Build history of the part. All positions in model axes, mm. A direction names the side the tool comes from. Give positions to 0.01 mm unless a question says otherwise; leave off trailing zeros. Loops run counter-clockwise (first coordinate to the right, second up) from the corner with the lowest first, then second, coordinate; pieces in that order, holes last.
1) Two-plate mould, pull along X, no slides. Class faces 1 (the cylindrical face through (23.09, -9.58, -15.04)), 2 (the flat face through (39, 0, -16)), 3 (the cylindrical face through (20.159, 25.743, -9.706)): +X half, -X half, draft (parallel to the pull), parting line (faces both ways), or undercut.
2) Band-saw the part on C-C on x = 46. List the corners of the cut face in (y, z).
3) Wall check: line 1 (Y direction, x = 0, z = -15.1); line 2 (Y direction, x = 0, z = -13.85); line 3 (X direction, y = -50, z = -14.75). Give the ranges that are in metal, low to high.
4) Band-saw the part on A-A on y = 0. List the corners of the cut face in (x, z).
5) Flat gauge pins, fed straight in: P1, Ø2, axis at x = 21, y = 33, coming from the -Z side; P2, Ø1.2, axis at y = -39.5, z = -15, coming from the +X side; P3, Ø8, axis at y = 41, z = -2, coming from the +X side; P4, Ø7, axis at x = 22.5, y = 22.5, coming from the +Z side. Where does each tip first touch, or does it go through?
6) 3-axis set-ups, long thin cutter, end or side, ignore diameter. For faces 4 (the flat face through (-21, 33, 0)), 5 (the conical face through (24.74, 7.79, -11.75)), 6 (the cylindrical face through (-8.67, -39.05, -4.06)): which of +Z, -Z, +X, -X, +Y, -Y reach the whole face in a straight line?
```python
from build123d import *

# Parameters (mm, degrees)
CYLINDER004_R     = 23.5
CYLINDER004_DEPTH = 6
CYLINDER003_R     = 25
CYLINDER003_DEPTH = 6
CYLINDER_R        = 4
CYLINDER_DEPTH    = 10
CYLINDER005_R     = 25
CYLINDER005_DEPTH = 6
BOX_W             = 110
BOX_H             = 18
BOX_DEPTH         = 1.5
BOX001_W          = 18
BOX001_H          = 110
BOX001_DEPTH      = 1.5
CYLINDER002_R     = 38.5
CYLINDER002_DEPTH = 8
CYLINDER001_R     = 40
CYLINDER001_DEPTH = 8


with BuildPart() as cilindro004:
    # Cylinder004 → Cylinder004 (new body)
    with BuildSketch(Plane.XY.offset(-18)):
        Circle(CYLINDER004_R)
    extrude(amount=CYLINDER004_DEPTH)


with BuildPart() as cut002:
    # Cylinder003 → Cylinder003 (new body)
    with BuildSketch(Plane.XY.offset(-18)):
        Circle(CYLINDER003_R)
    extrude(amount=CYLINDER003_DEPTH)

    # Cut002: cut Cilindro004
    add(cilindro004.part, mode=Mode.SUBTRACT)


with BuildPart() as cilindro:
    # Cylinder → Cylinder (new body)
    with BuildSketch(Plane(origin=(22.5, 22.5, -14), x_dir=(1, 0, 0), z_dir=(0, 0, 1))):
        Circle(CYLINDER_R)
    extrude(amount=CYLINDER_DEPTH)


with BuildPart() as cono001:
    # Cone001 → Cone001 (revolve)
    with BuildSketch(Plane(origin=(0, 0, -12), x_dir=(1, 0, 0), z_dir=(0, -1, 0))):
        Polygon((0, 0), (23.5, 0), (38.5, 4), (0, 4), align=None)
    revolve(axis=Axis((0, 0, -12), (0, 0, 1)))


with BuildPart() as cut004:
    # Cone → Cone (revolve)
    with BuildSketch(Plane(origin=(0, 0, -12), x_dir=(1, 0, 0), z_dir=(0, -1, 0))):
        Polygon((0, 0), (25, 0), (40, 4), (0, 4), align=None)
    revolve(axis=Axis((0, 0, -12), (0, 0, 1)))

    # Cut001: cut Cono001
    add(cono001.part, mode=Mode.SUBTRACT)

    # Cut004: cut Cilindro
    add(cilindro.part, mode=Mode.SUBTRACT)


with BuildPart() as cilindro005:
    # Cylinder005 → Cylinder005 (new body)
    with BuildSketch(Plane.XY.offset(-18)):
        Circle(CYLINDER005_R)
    extrude(amount=CYLINDER005_DEPTH)


with BuildPart() as cubo:
    # Box → Box (new body)
    with BuildSketch(Plane(origin=(-55, -9, 0), x_dir=(1, 0, 0), z_dir=(0, 0, 1))):
        with Locations((55, 9)):
            Rectangle(BOX_W, BOX_H)
    extrude(amount=BOX_DEPTH)


with BuildPart() as cut005:
    # Box001 → Box001 (new body)
    with BuildSketch(Plane(origin=(-9, -55, 0), x_dir=(1, 0, 0), z_dir=(0, 0, 1))):
        with Locations((9, 55)):
            Rectangle(BOX001_W, BOX001_H)
    extrude(amount=BOX001_DEPTH)

    # Fusion: union Cubo
    add(cubo.part)


with BuildPart() as cut005_1:
    # Fusion placement: moved
    add(cut005.part.moved(Location((0, 0, -16))))

    # Cut005: cut Cilindro005
    add(cilindro005.part, mode=Mode.SUBTRACT)


with BuildPart() as cilindro002:
    # Cylinder002 → Cylinder002 (new body)
    with BuildSketch(Plane.XY.offset(-8)):
        Circle(CYLINDER002_R)
    extrude(amount=CYLINDER002_DEPTH)


with BuildPart() as fusion001:
    # Cylinder001 → Cylinder001 (new body)
    with BuildSketch(Plane.XY.offset(-8)):
        Circle(CYLINDER001_R)
    extrude(amount=CYLINDER001_DEPTH)

    # Cut: cut Cilindro002
    add(cilindro002.part, mode=Mode.SUBTRACT)

    # Fusion001: union Cut002, Cut004, Cut005
    add(cut002.part)
    add(cut004.part)
    add(cut005_1.part)


solid = fusion001.part
```
Findings below:
1. face 1: parting line
1. face 2: draft
1. face 3: undercut
2. outline: (-9, -16) - (9, -16) - (9, -14.5) - (-9, -14.5) - close
3. line 1: y = -55 to -23.5, 23.5 to 55
3. line 2: y = -25 to -23.5, 23.5 to 25
3. line 3: x = -9 to 9
4. outline: (-55, -16) - (-25, -16) - (-25, -18) - (-23.5, -18) - (-23.5, -12) - (-38.5, -8) - (-38.5, 0) - (-40, 0) - (-40, -8) - (-25, -12) - (-25, -14.5) - (-55, -14.5) - close; (23.5, -18) - (25, -18) - (25, -16) - (55, -16) - (55, -14.5) - (25, -14.5) - (25, -12) - (40, -8) - (40, 0) - (38.5, 0) - (38.5, -8) - (23.5, -12) - close
5. P1: stops at z = -8.5
5. P2: stops at x = 9
5. P3: stops at x = 15.2
5. P4: passes through
6. face 4: +Z, +X, -X, +Y, -Y
6. face 5: none
6. face 6: +Z
